Job drawing, mm, ordinate dimensions from the low corner. One solid piece. Give positions to 0.01 mm unless a question says otherwise; leave off trailing zeros. Loops run counter-clockwise (first coordinate to the right, second up) from the corner with the lowest first, then second, coordinate; pieces in that order, holes last. Notation, with made-up numbers: M 26.5,47.5 L 42.5,47.5 A28 cw 42.5,85.5 Z; hole C 39.25,70.25 d11. An arc over 180 degrees is marked long. One line per question, with ' | ' between items.
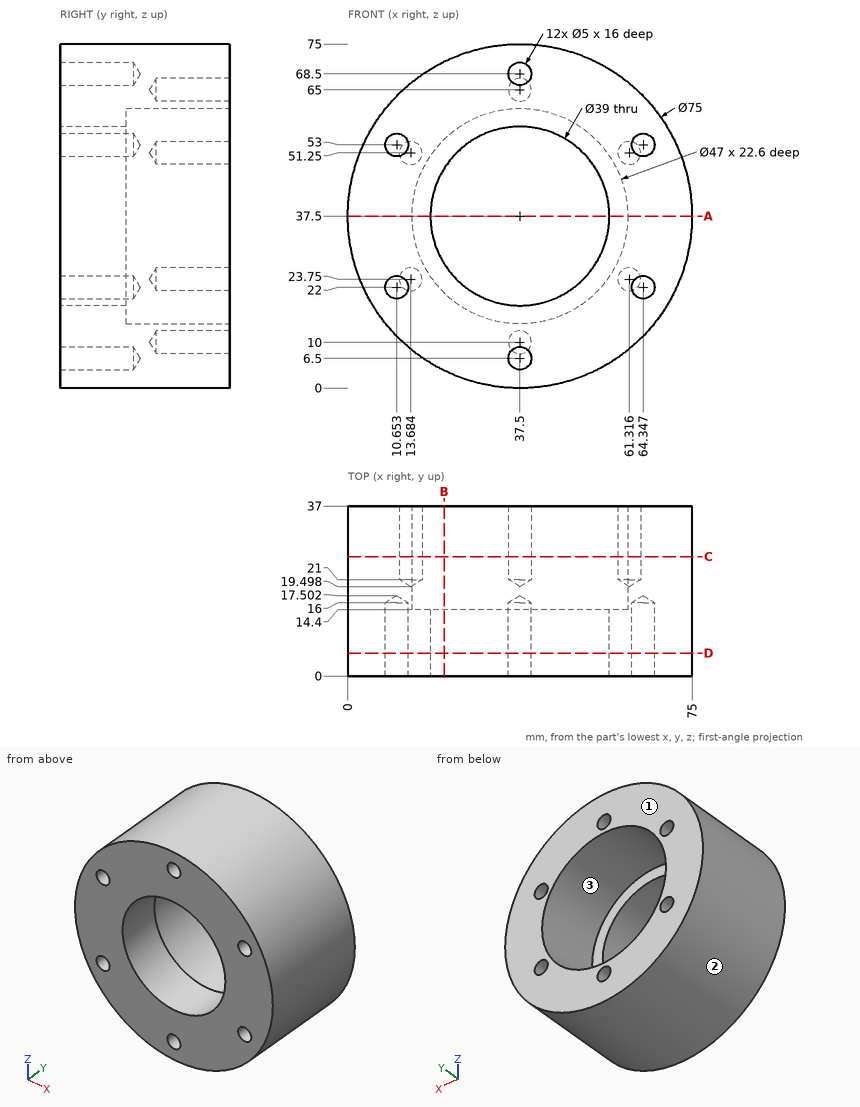
Item 1: Saw through at C-C on y = 26. Give the cut face in (x, z).
Conclusion:
outline: C 37.5,37.5 d75; hole C 13.68,23.75 d5; hole C 13.68,51.25 d5; hole C 37.5,37.5 d47; hole C 37.5,10 d5; hole C 37.5,65 d5; hole C 61.32,23.75 d5; hole C 61.32,51.25 d5
Item 2: Mould opens along Z. For the marked faces 1, 2 and 3 say: pulls with the +Z half, pulls with the -Z half, needs draft (parallel to the pull), parting line crosses it, or undercut.
Conclusion:
face 1: needs draft | face 2: parting line crosses it | face 3: undercut
Item 3: Saw through at A-A on z = 37.5. Give the cut face in (x, y), and give its area (3 significant figures).
Conclusion:
outline: M 0,0 L 18,0 L 18,14.4 L 14,14.4 L 14,37 L 0,37 Z; M 57,0 L 75,0 L 75,37 L 61,37 L 61,14.4 L 57,14.4 Z | area: 1,150 mm²
Item 4: Drop flat-ended pins along their axis: P1, Ø4, axis at x = 37.5, z = 65, coming from the +Y side; P2, Ø4.5, axis at x = 64.35, z = 53, coming from the -Y side; P3, Ø3, axis at x = 10.65, z = 53, coming from the -Y side. Give the stop position or say it passes through.
Conclusion:
P1: y = 20.7 | P2: y = 16.15 | P3: y = 16.6
Item 5: Saw through at D-D on y = 5. Give the cut face in (x, z).
Conclusion:
outline: C 37.5,37.5 d75; hole C 10.65,22 d5; hole C 10.65,53 d5; hole C 37.5,37.5 d39; hole C 37.5,6.5 d5; hole C 37.5,68.5 d5; hole C 64.35,22 d5; hole C 64.35,53 d5
Item 6: Drill centre lines: line 1 along Z through (x, y) = (37.5, 6.25); line 2 along Z through (x, y) = (37.5, 30.25); line 3 along X through (y, z) = (30.75, 23.75) (1 decimal). Where is each one in solid material? Low to high. Write a range as [from, to].
Conclusion:
line 1: [0, 4], [9, 18], [57, 66], [71, 75] | line 2: [0, 7.5], [12.5, 14], [61, 62.5], [67.5, 75] | line 3: [2.6, 11.2], [16.2, 18.4], [56.6, 58.8], [63.8, 72.4]
Item 7: Saw through at B-B on x = 21. Give the cut face in (y, z) (1 decimal), and give its area (3 significant figures).
Conclusion:
outline: M 0,3.8 L 37,3.8 L 37,20.8 L 14.4,20.8 L 14.4,27.1 L 0,27.1 Z; M 0,47.9 L 14.4,47.9 L 14.4,54.2 L 37,54.2 L 37,71.2 L 0,71.2 Z | area: 1,440 mm²
